Read the model definition and answer for the solid it produces. Units are mm, in the model's axes. Coordinates: 2 decimals unless noted, no trailing zeros. Loops run counter-clockwise (first coordinate to the right, second up) from the corner with the lowest first, then second, coordinate; pieces in that order, holes last. Notation, with made-up numbers: (-25, -32) - (-16, -32) arc R25 cw to (-16, -15) - close; hole circle Ø7 at (61.5, 42). An arc over 180 degrees is marked (long way). Use one line per item in the form item = value.
from build123d import *

# Parameters (mm, degrees)
SKETCH_1_R      = 1.75
SKETCH_1_R_2    = 3
EXTRUDE_2_DEPTH = 10


with BuildPart() as part:
    # 草图1 → 凸台-拉伸2 (new body)
    # profile 1 of 3: a face of its own
    with BuildSketch(Plane.XY):
        with BuildLine():
            Line((-46.972427161, 9.823182252), (-47.276428481, 9.823182252))
            ThreePointArc((-47.276428481, 9.823182252), (-54.622887383, 2.17272203), (-46.972427161, -5.173736872))
            ThreePointArc((-46.972427161, -5.173736872), (-41.767656174, -2.92456274), (-39.624427821, 2.32472269))
            ThreePointArc((-39.624427821, 2.32472269), (-41.767656174, 7.57400812), (-46.972427161, 9.823182252))
        make_face()
        with Locations((-47.124427821, 2.32472269)):
            Circle(SKETCH_1_R, mode=Mode.SUBTRACT)
    # profile 2 of 3: a face of its own
    with BuildSketch(Plane.XY):
        with BuildLine():
            Line((33.027572839, 9.823182252), (-46.972427161, 9.823182252))
            ThreePointArc((-46.972427161, 9.823182252), (-41.767656174, 7.57400812), (-39.624427821, 2.32472269))
            ThreePointArc((-39.624427821, 2.32472269), (-41.767656174, -2.92456274), (-46.972427161, -5.173736872))
            Line((-46.972427161, -5.173736872), (33.027572839, -5.173736872))
            ThreePointArc((33.027572839, -5.173736872), (25.679573499, 2.32472269), (33.027572839, 9.823182252))
        make_face()
    # profile 3 of 3: a face of its own
    with BuildSketch(Plane.XY):
        with BuildLine():
            Line((33.331574159, 9.823182252), (33.027572839, 9.823182252))
            ThreePointArc((33.027572839, 9.823182252), (25.679573499, 2.32472269), (33.027572839, -5.173736872))
            ThreePointArc((33.027572839, -5.173736872), (38.428858929, -3.032048957), (40.679573499, 2.32472269))
            ThreePointArc((40.679573499, 2.32472269), (38.536345146, 7.57400812), (33.331574159, 9.823182252))
        make_face()
        with Locations((33.179573499, 2.32472269)):
            Circle(SKETCH_1_R_2, mode=Mode.SUBTRACT)
    extrude(amount=EXTRUDE_2_DEPTH)


solid = part.part
Item 1: This flat-tipped pin is pushed along its axis until it touches: P1, Ø2, axis at y = 1, z = 7, coming from the -X side. Where does it stop, or does it pass through?
Results below:
P1 = -54.62
Item 2: For a pull along X with two mould halves and no side action, classify faces 1 (the flat face through (-6, 9.823, 5)), 2 (the cylindrical face through (30.182, 2.457, 4.93)) as +X half, -X half, draft (parallel to the pull), parting line (faces both ways), or undercut.
Results below:
face_1 = draft
face_2 = undercut
Item 3: Find the intervals of material crossed by L1, parallel to X at y = 2, z = 5.25; L2, parallel to X at y = 0.75, z = 3.25; L3, parallel to Y at x = 22, z = 3.5, in increasing order.
Results below:
L1 = -54.62 to -48.84, -45.4 to 30.2, 36.16 to 40.67
L2 = -54.46 to -47.89, -46.36 to 30.63, 35.73 to 40.51
L3 = -5.17 to 9.82
Item 4: The part is cut by section B-B on y = 1.5. Give the vertices of the cut face in (x, z), plus the area to 3 significant figures.
Results below:
outline = (-54.58, 0) - (-48.67, 0) - (-48.67, 10) - (-54.58, 10) - close; (-45.58, 0) - (30.3, 0) - (30.3, 10) - (-45.58, 10) - close; (36.06, 0) - (40.63, 0) - (40.63, 10) - (36.06, 10) - close
area = 864 mm²
Item 5: The part is cut by section D-D on y = 7. Give the vertices of the cut face in (x, z), plus the area to 3 significant figures.
Results below:
outline = (-52.99, 0) - (39.04, 0) - (39.04, 10) - (-52.99, 10) - close
area = 920 mm²
Item 6: The part is cut by section C-C on y = -3.25. Give the vertices of the cut face in (x, z).
Results below:
outline = (-52.14, 0) - (38.2, 0) - (38.2, 10) - (-52.14, 10) - close
